The listing builds one solid part. Answer for the finished solid, in the listing's coordinates (mm). A direction names the side the tool comes from. Coordinates: 2 decimals unless noted, no trailing zeros. Write each loop counter-clockwise with the first axis right and the second up, starting at its lowest first coordinate (ties: lowest second). Pieces come first, ordered by that corner, then holes.
Autodesk Inventor part; units mm, degrees
ref_plane "YZ Plane" through (0, 0, 0) normal (1, 0, 0) x (0, 1, 0)
ref_plane "XZ Plane" through (0, 0, 0) normal (0, 1, 0) x (-1, 0, 0)
ref_plane "XY Plane" through (0, 0, 0) normal (0, 0, 1) x (1, 0, 0)
sketch "Esboço1" plane through (0, 0, 0) normal (0, 0, 1) x (1, 0, 0)
  line L0 (1.0341, 28.7122) -> (1.0341, -32.1101) construction
  line L1 (1.0341, 7.7011) -> (-4.7241, 7.7011)
  line L2 (-4.7241, 7.7011) -> (-6.4659, 5.9592)
  line L3 (-6.4659, 5.9592) -> (-6.4659, 3.9592)
  line L4 (-6.4659, 3.9592) -> (-5.2631, 2.7564)
  line L5 (-5.2631, 2.7564) -> (-5.2631, -0.2436)
  line L6 (-5.2631, -0.2436) -> (-6.4659, -1.4465)
  line L7 (-6.4659, -1.4465) -> (-6.4659, -1.6989)
  line L8 (-6.4659, -6.2989) -> (1.0341, -6.2989) construction
  line L9 (-22.4659, 9.7011) -> (-22.4659, 17.7011)
  line L10 (-17.9659, 24.9392) -> (-17.9659, -12.707) construction
  line L11 (-20.4659, 24.9392) -> (-20.4659, -12.707) construction
  line L12 (-15.4659, 24.9392) -> (-15.4659, -12.9196) construction
  line L13 (1.0341, 9.7011) -> (-29.6062, 9.7011) construction
  line L14 (-22.4659, 9.7011) -> (-14.8619, 9.7011)
  line L15 (-14.8619, 9.7011) -> (-14.8619, -1.6989)
  line L16 (1.0341, 16.4633) -> (-13.4863, 16.4633) construction
  line L17 (-13.4863, 16.4633) -> (-13.4863, -1.6989) construction
  arc A0 (-14.8619, -1.6989) -> (-22.4659, 9.7011) centre (-28.6186, -2.6389) ccw construction
  line L18 (-6.4659, -1.6989) -> (-6.4659, -6.2989) construction
  line L19 (-6.4659, -1.6989) -> (-14.8619, -1.6989)
  line L20 (-13.4863, 17.7011) -> (-12.9262, 17.1409)
  line L21 (-12.9262, 17.1409) -> (-5.8645, 17.1409)
  line L22 (-5.8645, 17.1409) -> (-5.3043, 17.7011)
  line L23 (-22.4659, 17.7011) -> (-13.4863, 17.7011)
  line L24 (-5.3043, 17.7011) -> (1.0341, 17.7011)
  line L25 (1.0341, 7.7011) -> (6.7923, 7.7011)
  line L26 (6.7923, 7.7011) -> (8.5341, 5.9592)
  line L27 (8.5341, 5.9592) -> (8.5341, 3.9592)
  line L28 (8.5341, 3.9592) -> (7.3313, 2.7564)
  line L29 (7.3313, 2.7564) -> (7.3313, -0.2436)
  line L30 (7.3313, -0.2436) -> (8.5341, -1.4465)
  line L31 (8.5341, -1.4465) -> (8.5341, -1.6989)
  line L32 (8.5341, -6.2989) -> (1.0341, -6.2989) construction
  line L33 (24.5341, 9.7011) -> (24.5341, 17.7011)
  line L34 (20.0341, 24.9392) -> (20.0341, -12.707) construction
  line L35 (22.5341, 24.9392) -> (22.5341, -12.707) construction
  line L36 (17.5341, 24.9392) -> (17.5341, -12.9196) construction
  line L37 (1.0341, 9.7011) -> (31.6744, 9.7011) construction
  line L38 (24.5341, 9.7011) -> (16.9301, 9.7011)
  line L39 (16.9301, 9.7011) -> (16.9301, -1.6989)
  line L40 (1.0341, 16.4633) -> (15.5546, 16.4633) construction
  line L41 (15.5546, 16.4633) -> (15.5546, -1.6989) construction
  arc A1 (24.5341, 9.7011) -> (16.9301, -1.6989) centre (30.6868, -2.6389) ccw construction
  line L42 (8.5341, -1.6989) -> (8.5341, -6.2989) construction
  line L43 (8.5341, -1.6989) -> (16.9301, -1.6989)
  line L44 (15.5546, 17.7011) -> (14.9944, 17.1409)
  line L45 (14.9944, 17.1409) -> (7.9327, 17.1409)
  line L46 (7.9327, 17.1409) -> (7.3725, 17.7011)
  line L47 (24.5341, 17.7011) -> (15.5546, 17.7011)
  line L48 (7.3725, 17.7011) -> (1.0341, 17.7011)
  dimension "d11" = 45
  dimension "d12" = 3
  dimension "d13" = 14
  dimension "d14" = 2
  dimension "d15" = 7.5
  dimension "d19" = 23.5
  dimension "d21" = 2.5
  dimension "d22" = 2.5
  dimension "d23" = 19
extrude "Extrusão2" add sketch "Esboço1" along normal blind 40
sketch "Esboço2" plane through (0, 0, 40) normal (0, 0, 1) x (1, 0, 0)
  line L0 (-13.0314, -1.4465) -> (-13.0314, 15.7348)
  line L1 (-13.0314, 15.7348) -> (15.0996, 15.7348)
  line L2 (15.0996, 15.7348) -> (15.0996, -1.4465)
  line L3 (-6.4659, -1.4465) -> (-5.2631, -0.2436)
  line L4 (-6.4659, -1.4465) -> (-5.2631, -0.2436)
  line L5 (-5.2631, 2.7564) -> (-6.4659, 3.9592)
  line L6 (-5.2631, -0.2436) -> (-5.2631, 2.7564)
  line L7 (-5.2631, 2.7564) -> (-6.4659, 3.9592)
  line L8 (-6.4659, 3.9592) -> (-6.4659, 5.9592)
  line L9 (-6.4659, 3.9592) -> (-6.4659, 5.9592)
  line L10 (-6.4659, 5.9592) -> (-4.7241, 7.7011)
  line L11 (-6.4659, 5.9592) -> (-4.7241, 7.7011)
  line L12 (-4.7241, 7.7011) -> (6.7923, 7.7011)
  line L13 (-4.7241, 7.7011) -> (6.7923, 7.7011)
  line L14 (6.7923, 7.7011) -> (8.5341, 5.9592)
  line L15 (6.7923, 7.7011) -> (8.5341, 5.9592)
  line L16 (8.5341, 3.9592) -> (8.5341, 5.9592)
  line L17 (8.5341, 5.9592) -> (8.5341, 3.9592)
  line L18 (7.3313, -0.2436) -> (7.3313, 2.7564)
  line L19 (8.5341, 3.9592) -> (7.3313, 2.7564)
  line L20 (7.3313, 2.7564) -> (7.3313, -0.2436)
  line L21 (8.5341, -1.4465) -> (7.3313, -0.2436)
  line L22 (7.3313, -0.2436) -> (8.5341, -1.4465)
  line L23 (15.0996, -1.4465) -> (8.5341, -1.4465)
  line L24 (-6.4659, -1.4465) -> (-13.0314, -1.4465)
extrude "Extrusão3" add sketch "Esboço2" along normal blind 7.5
sketch "Esboço3" plane through (0, 0, 0) normal (0, 0, -1) x (-1, 0, 0)
  line L0 (-15.0996, -1.4465) -> (-15.0996, 15.7348)
  line L1 (-15.0996, 15.7348) -> (13.0314, 15.7348)
  line L2 (13.0314, 15.7348) -> (13.0314, -1.4465)
  line L3 (-8.5341, -1.4465) -> (-7.3313, -0.2436)
  line L4 (-8.5341, -1.4465) -> (-7.3313, -0.2436)
  line L5 (-7.3313, 2.7564) -> (-8.5341, 3.9592)
  line L6 (-7.3313, -0.2436) -> (-7.3313, 2.7564)
  line L7 (-7.3313, 2.7564) -> (-8.5341, 3.9592)
  line L8 (-8.5341, 3.9592) -> (-8.5341, 5.9592)
  line L9 (-8.5341, 3.9592) -> (-8.5341, 5.9592)
  line L10 (-8.5341, 5.9592) -> (-6.7923, 7.7011)
  line L11 (-8.5341, 5.9592) -> (-6.7923, 7.7011)
  line L12 (-6.7923, 7.7011) -> (4.7241, 7.7011)
  line L13 (-6.7923, 7.7011) -> (4.7241, 7.7011)
  line L14 (4.7241, 7.7011) -> (6.4659, 5.9592)
  line L15 (4.7241, 7.7011) -> (6.4659, 5.9592)
  line L16 (6.4659, 3.9592) -> (6.4659, 5.9592)
  line L17 (6.4659, 5.9592) -> (6.4659, 3.9592)
  line L18 (5.2631, -0.2436) -> (5.2631, 2.7564)
  line L19 (6.4659, 3.9592) -> (5.2631, 2.7564)
  line L20 (5.2631, 2.7564) -> (5.2631, -0.2436)
  line L21 (6.4659, -1.4465) -> (5.2631, -0.2436)
  line L22 (5.2631, -0.2436) -> (6.4659, -1.4465)
  line L23 (13.0314, -1.4465) -> (6.4659, -1.4465)
  line L24 (-8.5341, -1.4465) -> (-15.0996, -1.4465)
  point P0 (0, 0)
  point P1 (-1.0341, 15.7348)
extrude "Extrusão4" add sketch "Esboço3" along normal blind 7.5
sketch "Esboço4" plane through (-5.3043, 17.7011, 0) normal (0, 1, 0) x (1, 0, 0)
  line L0 (6.3384, -52.3357) -> (6.3384, 13.624) construction
  line L1 (-22.2826, -19.2901) -> (34.758, -19.2901) construction
  circle A0 centre (-12.6616, -34.2901) radius 1 construction
  circle A1 centre (-12.6616, -4.2901) radius 1 construction
  circle A2 centre (25.3384, -34.2901) radius 1 construction
  circle A3 centre (25.3384, -4.2901) radius 1 construction
  dimension "d31" = 2
  dimension "d32" = 2
  dimension "d33" = 2
  dimension "d34" = 2
  dimension "d35" = 19
  dimension "d36" = 19
  dimension "d37" = 19
  dimension "d38" = 19
  dimension "d39" = 15
  dimension "d40" = 15
  dimension "d41" = 15
  dimension "d42" = 15
hole "Furo1" at (-17.9659, 17.7011, 4.2901) at (-17.9659, 17.7011, 34.2901) at (20.0341, 17.7011, 34.2901) at (20.0341, 17.7011, 4.2901) direction (0, -1, 0) diameter 4.134 end through all
equation "\"d22\" = d21"
equation "\"d36\" = d35"
equation "\"d37\" = d35"
equation "\"d38\" = d35"
equation "\"d40\" = d39"
equation "\"d41\" = d39"
equation "\"d42\" = d39"
properties part number "PATINS TRILHO LINEAR 15MM DFH-A_AL"
1. Section A-A on y = 0.5 is taken. Give the vertices of the cut face in (x, z), then the cut area to 3 significant figures.
Results found:
outline: (-14.86, 0) - (-13.03, 0) - (-13.03, -7.5) - (-5.26, -7.5) - (-5.26, 47.5) - (-13.03, 47.5) - (-13.03, 40) - (-14.86, 40) - close; (7.33, -7.5) - (15.1, -7.5) - (15.1, 0) - (16.93, 0) - (16.93, 40) - (15.1, 40) - (15.1, 47.5) - (7.33, 47.5) - close
area: 1,000 mm2
2. Section B-B on x = -2.5 is taken. Give the vertices of the cut face in (y, z).
Results found:
outline: (7.7, -7.5) - (15.73, -7.5) - (15.73, 0) - (17.7, 0) - (17.7, 40) - (15.73, 40) - (15.73, 47.5) - (7.7, 47.5) - close
3. Section C-C on y = 9 is taken. Give the vertices of the cut face in (x, z), then the cut area to 3 significant figures.
Results found:
outline: (-14.86, 0) - (-13.03, 0) - (-13.03, -7.5) - (15.1, -7.5) - (15.1, 0) - (16.93, 0) - (16.93, 40) - (15.1, 40) - (15.1, 47.5) - (-13.03, 47.5) - (-13.03, 40) - (-14.86, 40) - close
area: 1,690 mm2
4. A tool of negligible diameter and unlimited length cuts with its end or side. For faces 4 (the flat face through (12, -1.446, 44)), 5 (the flat face through (1, 15.735, 44)), 6 (the flat face through (12, 17.141, 20)), 7 (the flat face through (7.331, 1, 20)), from which of +Z, -Z, +X, -X, +Y, -Y can it reach the whole face along a straight path? Write none if from no direction.
Results found:
face 4: +Z, +X, -X, -Y
face 5: +Z, +X, -X, +Y
face 6: +Z, -Z, +Y
face 7: +Z, -Z, -Y
5. Find the intervals of material crossed by L1, parallel to X at y = 5, z = 38; L2, parallel to X at y = 1.75, z = 12; L3, parallel to Y at x = -2, z = 38, in increasing order.
Results found:
L1: x = -14.86 to -6.47, 8.53 to 16.93
L2: x = -14.86 to -5.26, 7.33 to 16.93
L3: y = 7.7 to 17.7
6. Flat-ended cylindrical pins translate along their axes: P1, Ø5.5, axis at y = 1.5, z = 18.5, coming from the +X side; P2, Ø7, axis at x = 10.5, z = 45.5, coming from the -Y side; P3, Ø2, axis at x = -10, z = 19, coming from the +Y side; P4, Ø12, axis at x = 20, z = -1, coming from the -Y side. Find the tip coordinate at first contact, or state that the pin passes through.
Results found:
P1: stops at x = 16.93
P2: stops at y = -1.45
P3: stops at y = 17.14
P4: stops at y = -1.7
7. For a pull along X with two mould halves and no side action, classify faces 1 (the flat face through (7.94, -0.85, 20.39)), 2 (the flat face through (-22.466, 14, 20)), 3 (the flat face through (-10, -1.446, -4)) as pulls with the +X half, pulls with the -X half, needs draft (parallel to the pull), parting line crosses it, or undercut.
Results found:
face 1: undercut
face 2: pulls with the -X half
face 3: needs draft
